Read the model definition and answer for the solid it produces. Units are mm, in the model's axes. A direction names the side the tool comes from. Give positions to 0.01 mm unless a question says otherwise; leave off trailing zeros. Order: outer loops, then holes, each group sorted by start corner. A loop starts at its lowest first (then second) coordinate and runs counter-clockwise, first axis right, second up. Notation, with made-up numbers: (53, 71) - (106, 71) arc R33 cw to (106, 102) - close; hole circle Ø8 at (42.5, -28). An arc over 180 degrees is marked (long way). Use a Markdown table: item, result. Add a question column.
1. For a pull along X with two mould halves and no side action, classify faces 1 (the flat face through (-1, -6, 2)), 2 (the cylindrical face through (3.81, -104.93, 0.99)), 3 (the cylindrical face through (42.3, 68.8, 1)) as released by +X, released by -X, zero draft, split by the parting line, or undercut.
2. Which of the six approach directions +Z, -Z, +X, -X, +Y, -Y give full straight-line access (tool end or side, diameter ignored) to faces 4 (the flat face through (-1, -6, 0)), 5 (the cylindrical face through (-41.8, 68.4, 1))?
3. A cutting plane is placed at A-A on y = 25.5. Determine the outline of the cut face in (x, z), and give its area (3 significant figures).
4. Flat-ended cylindrical pins translate along their axes: P1, Ø2.5, axis at x = 0, y = 0, coming from the -Z side; P2, Ø1, axis at x = 39, z = 1, coming from the -Y side; P3, Ø1, axis at y = 18, z = 0.5, coming from the +X side. Find the tip coordinate at first contact, or state that the pin passes through.
5. A cutting plane is placed at B-B on z = 0.45. State how many separate pieces and enclosed holes the cut face has, and give its area (3 significant figures).
6. A cutting plane is placed at D-D on y = -55.5. Determine the outline of the cut face in (x, z), and give its area (3 significant figures).
7. Consider L1, parallel to X at y = 15, z = 0.5; L2, parallel to X at y = -86, z = 1.15; L3, parallel to Y at x = -33.5, z = 1.2. Determine where each line is inside the solid, lowest interval first.
8. A cutting plane is placed at C-C on x = 78.5. Determine the outline of the cut face in (y, z).
Autodesk Inventor part; units mm, degrees
ref_plane "YZ Plane" through (0, 0, 0) normal (1, 0, 0) x (0, 1, 0)
ref_plane "XZ Plane" through (0, 0, 0) normal (0, 1, 0) x (-1, 0, 0)
ref_plane "XY Plane" through (0, 0, 0) normal (0, 0, 1) x (1, 0, 0)
sketch "Skizze3" plane through (0, 0, 0) normal (0, 0, 1) x (1, 0, 0)
  arc A0 (-55.0029, 89.4409) -> (55.0029, 89.4409) centre (0, 0) ccw
  line L0 (0, 0) -> (55.0029, 89.4409) construction
  line L1 (0, 0) -> (105, 0) construction
  line L2 (0, 0) -> (-55.0029, 89.4409) construction
  line L3 (-55.0029, 89.4409) -> (-18.8829, 89.4409)
  line L4 (-18.8829, 89.4409) -> (-18.8829, 97.4409)
  arc A1 (-55.0029, 89.4409) -> (-18.8829, 60.4456) centre (-18.8829, 97.4409) ccw
  line L5 (55.0029, 89.4409) -> (18.8829, 89.4409)
  line L6 (18.8829, 89.4409) -> (18.8829, 97.4409)
  arc A2 (18.8839, 60.4456) -> (55.0029, 89.4409) centre (18.8829, 97.4409) ccw
  line L7 (18.8829, 97.4409) -> (18.8839, 60.4456) construction
  line L8 (18.8829, 97.4409) -> (55.0029, 89.4409) construction
  line L9 (-18.8829, 60.4456) -> (18.8839, 60.4456)
  line L10 (0, 0) -> (57.2785, 0) construction
  line L11 (0, 0) -> (57.2785, 0) construction
  line L12 (0, 0) -> (57.279, 0) construction
  line L13 (0, 0) -> (84.4383, 0) construction
  line L14 (0, 0) -> (90, 0) construction
  line L15 (0, 0) -> (90, 0) construction
  line L16 (0, 0) -> (90, 0) construction
  line L17 (0, 0) -> (97, 0) construction
  line L18 (0, 0) -> (97, 0) construction
  line L19 (0, 0) -> (97, 0) construction
  line L20 (0, 0) -> (97, 0) construction
  line L21 (0, 0) -> (100, 0) construction
  circle A3 centre (-93.9693, -34.202) radius 1.5
  line L22 (0, 0) -> (100, 0) construction
  line L23 (0, 0) -> (100, 0) construction
  line L24 (0, 0) -> (100, 0) construction
  circle A4 centre (-50, -86.6025) radius 1.5
  circle A5 centre (93.9693, -34.202) radius 1.5
  circle A6 centre (50, -86.6025) radius 1.5
  line L25 (0, 0) -> (100, 0) construction
  line L26 (0, 0) -> (100, 0) construction
  circle A7 centre (-64.2788, 76.6044) radius 1.5
  circle A8 centre (64.2788, 76.6044) radius 1.5
  line L27 (0, 0) -> (42, 0) construction
  line L28 (0, 0) -> (42, 0) construction
  circle A9 centre (-32.5, 56.2917) radius 1.5
  circle A10 centre (32.5, 56.2917) radius 1.5
  line L29 (-32.5, 56.2917) -> (32.5, 56.2917) construction
  line L30 (-32.5, 56.2917) -> (0, 0) construction
  line L31 (32.5, 56.2917) -> (0, 0) construction
  line L32 (0, 0) -> (0, -73.5) construction
  line L33 (0, -73.5) -> (-19, -73.5) construction
  circle A11 centre (-19, -73.5) radius 1.5
  line L34 (0, 0) -> (-64.2788, 76.6044) construction
  line L35 (0, 0) -> (100, 0) construction
  line L36 (0, 0) -> (64.2788, 76.6044) construction
  line L37 (0, 0) -> (100, 0) construction
  line L38 (0, 0) -> (-93.9693, -34.202) construction
  line L39 (0, 0) -> (100, 0) construction
  line L40 (0, 0) -> (93.9693, -34.202) construction
  line L41 (0, 0) -> (100, 0) construction
  line L42 (0, 0) -> (-50, -86.6025) construction
  line L43 (0, 0) -> (100, 0) construction
  line L44 (0, 0) -> (50, -86.6025) construction
  line L45 (0, 0) -> (100, 0) construction
  circle A12 centre (19, -73.5) radius 1.5
  line L46 (0, 0) -> (63.6529, 36.75) construction
  line L47 (0, 0) -> (73.5, 0) construction
  line L48 (63.6529, 36.75) -> (54.1529, 53.2045) construction
  circle A13 centre (54.1529, 53.2045) radius 1.5
  circle A14 centre (73.1529, 20.2955) radius 1.5
  circle A15 centre (-54.1529, 53.2045) radius 1.5
  circle A16 centre (-73.1529, 20.2955) radius 1.5
  circle A17 centre (0, 0) radius 1.5
  dimension "d22" = 105
  dimension "d23" = 58.41
  dimension "d24" = 63.18
  dimension "d25" = 36.12
  dimension "d26" = 8
  dimension "d27" = 90
  dimension "d28" = 36.12
  dimension "d29" = 8
  dimension "d30" = 90
  dimension "d31" = 77.51
  dimension "d140" = 3
  dimension "d153" = 65
  dimension "d154" = 120
  dimension "d163" = 60
  dimension "d172" = 73.5
  dimension "d173" = 19
  dimension "d174" = 100
  dimension "d175" = 130
  dimension "d176" = 100
  dimension "d177" = 50
  dimension "d178" = 100
  dimension "d179" = 160
  dimension "d180" = 100
  dimension "d181" = 20
  dimension "d182" = 100
  dimension "d183" = 120
  dimension "d184" = 100
  dimension "d185" = 60
  dimension "d186" = 73.5
  dimension "d187" = 30
  dimension "d188" = 19
  dimension "d189" = 3
extrude "Extrusion3" add sketch "Skizze3" along normal blind 2
sketch "Skizze5" plane through (0, 0, 2) normal (0, 0, 1) x (1, 0, 0)
  line L0 (-40, 19.2917) -> (40, 19.2917)
  line L1 (40, 19.2917) -> (40, 47.2917)
  line L2 (40, 47.2917) -> (-40, 47.2917)
  line L3 (-40, 47.2917) -> (-40, 19.2917)
  line L4 (0, 0) -> (0, 47.2917) construction
  line L5 (-37.5, 47.2917) -> (-27.5, 47.2917)
  line L6 (-27.5, 47.2917) -> (-27.5, 49.2917)
  line L7 (-27.5, 49.2917) -> (-37.5, 49.2917)
  line L8 (-37.5, 49.2917) -> (-37.5, 47.2917)
  line L9 (-40, 33.2917) -> (40, 33.2917) construction
  line L10 (-37.5, 19.2917) -> (-27.5, 19.2917)
  line L11 (-27.5, 19.2917) -> (-27.5, 17.2917)
  line L12 (-27.5, 17.2917) -> (-37.5, 17.2917)
  line L13 (-37.5, 17.2917) -> (-37.5, 19.2917)
  line L14 (37.5, 47.2917) -> (27.5, 47.2917)
  line L15 (27.5, 47.2917) -> (27.5, 49.2917)
  line L16 (27.5, 49.2917) -> (37.5, 49.2917)
  line L17 (37.5, 49.2917) -> (37.5, 47.2917)
  line L18 (37.5, 19.2917) -> (27.5, 19.2917)
  line L19 (27.5, 19.2917) -> (27.5, 17.2917)
  line L20 (27.5, 17.2917) -> (37.5, 17.2917)
  line L21 (37.5, 17.2917) -> (37.5, 19.2917)
  circle A0 centre (-32.5, 14.2917) radius 1.5
  circle A1 centre (32.5, 14.2917) radius 1.5
  circle A2 centre (-32.5, 56.2917) radius 1.5
  line L22 (-32.5, 49.2917) -> (-32.5, 56.2917) construction
  dimension "d158" = 80
  dimension "d159" = 28
  dimension "d164" = 10
  dimension "d165" = 2
  dimension "d169" = 3
  dimension "d171" = 7
extrude "Extrusion4" cut sketch "Skizze5" against normal up to next
properties part number "Hauptplatine" material "Kupfer"
Output values:
| question | item | result |
|---|---|---|
| 1 | face 1 | zero draft |
| 1 | face 2 | split by the parting line |
| 1 | face 3 | undercut |
| 2 | face 4 | -Z, +X, -X, +Y, -Y |
| 2 | face 5 | +Z, -Z, +Y |
| 3 | outline | (-101.86, 0) - (-40, 0) - (-40, 2) - (-101.86, 2) - close; (40, 0) - (101.86, 0) - (101.86, 2) - (40, 2) - close |
| 3 | area | 247 mm² |
| 4 | P1 | through |
| 4 | P2 | y = -97.69 |
| 4 | P3 | x = 103.53 |
| 5 | separate pieces | 1 |
| 5 | enclosed holes | 18 |
| 5 | area | 28,400 mm² |
| 6 | outline | (-89.13, 0) - (89.13, 0) - (89.13, 2) - (-89.13, 2) - close |
| 6 | area | 357 mm² |
| 7 | L1 | -103.92 to -33.82, -31.18 to 31.18, 33.82 to 103.92 |
| 7 | L2 | -60.24 to -51.37, -48.63 to 48.63, 51.37 to 60.24 |
| 7 | L3 | -99.51 to 13.17, 15.41 to 17.29, 49.29 to 55.17, 57.41 to 63.46 |
| 8 | outline | (-69.73, 0) - (69.73, 0) - (69.73, 2) - (-69.73, 2) - close |
